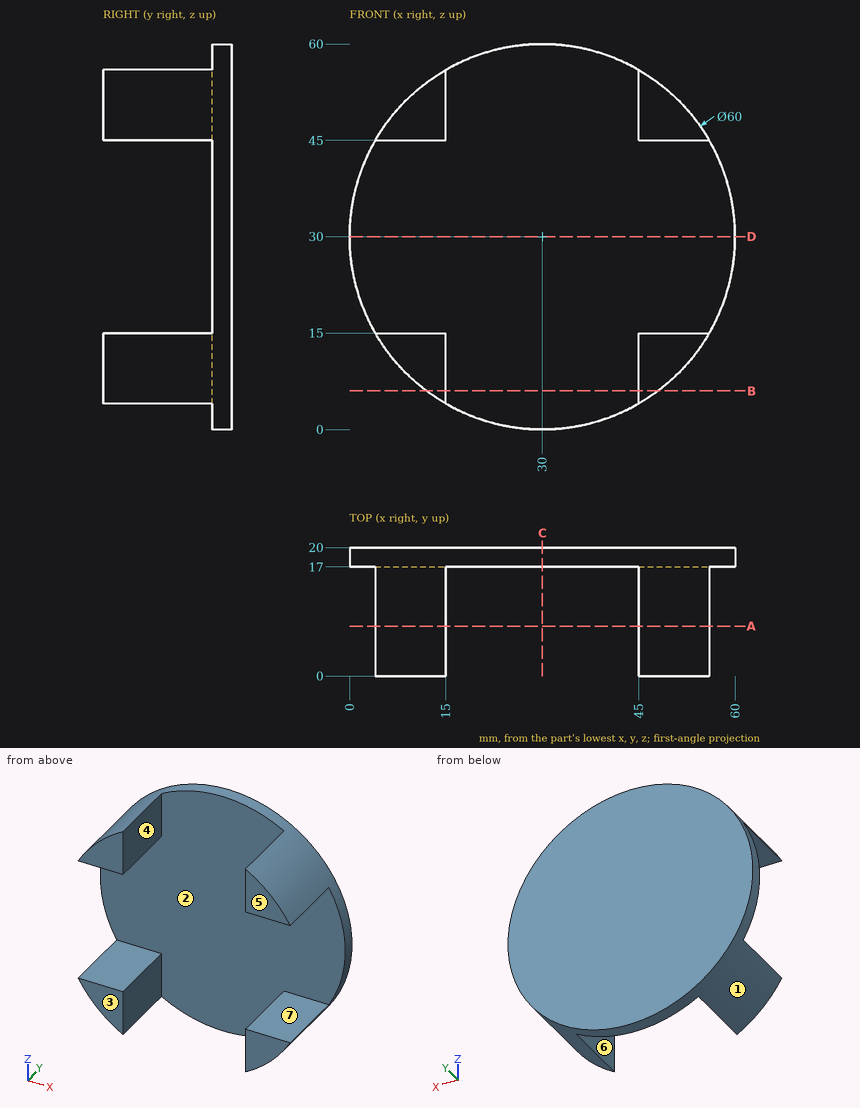
For this review, use the dimensioned drawing (mm, ordinates from the lowest corner) and the shaded views. A direction names the side the tool comes from. Coordinates: 2 decimals unless noted, no trailing zeros. Loops run counter-clockwise (first coordinate to the right, second up) from the corner with the lowest first, then second, coordinate; pieces in that order, holes last. Notation, with made-up numbers: M -21.75,55 L -17.75,55 A13 cw -17.75,74 Z; hole C -29.5,43.25 d3. An arc over 180 degrees is marked long. Answer as CSV lines item,"result".
Item 1: Add section B-B on z = 6. State the section outline as (x, y) points.
Answer list:
outline,"M 12,0 L 15,0 L 15,17 L 45,17 L 45,0 L 48,0 L 48,20 L 12,20 Z"
Item 2: Machinability: for the marked faces 5, 6 and 7, which of the approach directions +Z, -Z, +X, -X, +Y, -Y give a long, thin tool a straight path to every point of the face, cutting with its end or side? Answer none if there is none.
Answer list:
face 5,"+Z, -Z, +X, -X, -Y"
face 6,"+Z, -Z, -Y"
face 7,"+X, -X, -Y"
Item 3: Add section D-D on z = 30. State the section outline as (x, y) points.
Answer list:
outline,"M 0,17 L 60,17 L 60,20 L 0,20 Z"
Item 4: For P1, Ø1, axis at x = 7, z = 27.5, coming from the -Y side; P2, Ø5.5, axis at x = 9.5, y = 6, coming from the -Z side; P3, Ø5, axis at x = 43, y = 9.5, coming from the -Z side; P4, Ø1, axis at x = 52, z = 11.5, coming from the -Y side, all flat-tipped, find the tip position at first contact; note any pin that passes through.
Answer list:
P1,"y = 17"
P2,"z = 5.81"
P3,"z = 4.02"
P4,"y = 0"
Item 5: The part is to be moulded in two halves that separate along X. For the marked faces 1, 2, 3 and 4, say which applies: pulls with the +X half, pulls with the -X half, needs draft (parallel to the pull), parting line crosses it, or undercut.
Answer list:
face 1,"parting line crosses it"
face 2,"undercut"
face 3,"needs draft"
face 4,"undercut"
Item 6: Add section C-C on x = 30. State the section outline as (y, z) points.
Answer list:
outline,"M 17,0 L 20,0 L 20,60 L 17,60 Z"
Item 7: Add section A-A on y = 7.75. State the section outline as (x, z) points, plus the area to 3 significant figures.
Answer list:
outline,"M 4.02,15 A30 ccw 15,4.02 L 15,15 Z; M 4.02,45 L 15,45 L 15,55.98 A30 ccw Z; M 45,4.02 A30 ccw 55.98,15 L 45,15 Z; M 45,45 L 55.98,45 A30 ccw 45,55.98 Z"
area,"284 mm²"
Item 8: For probe 1 along Y at (x, z) = (24, 55); probe 2 along X at (y, z) = (11.75, 7); probe 3 along X at (y, z) = (3.75, 5.5), list the stretches that pass through material, from the lowest coordinate up.
Answer list:
probe 1,"17 to 20"
probe 2,"10.74 to 15, 45 to 49.26"
probe 3,"12.69 to 15, 45 to 47.31"
